Geometry: see drawing. Coordinates: mm, zero at the bounding-box minimum. Round coordinates to 2 decimals unless told otherwise and drop trailing zeros. Loops run counter-clockwise (first coordinate to the right, second up) from the corner with the lowest first, then second, coordinate; pieces in that order, holes last. Notation, with made-up numbers: (41, 39) - (86, 39) arc R25 ccw to (86, 58) - close; hole circle Ø4 at (24.5, -35). An arc over 180 degrees is marked (long way). Use CSV: the item, a comma, the result in double quotes.
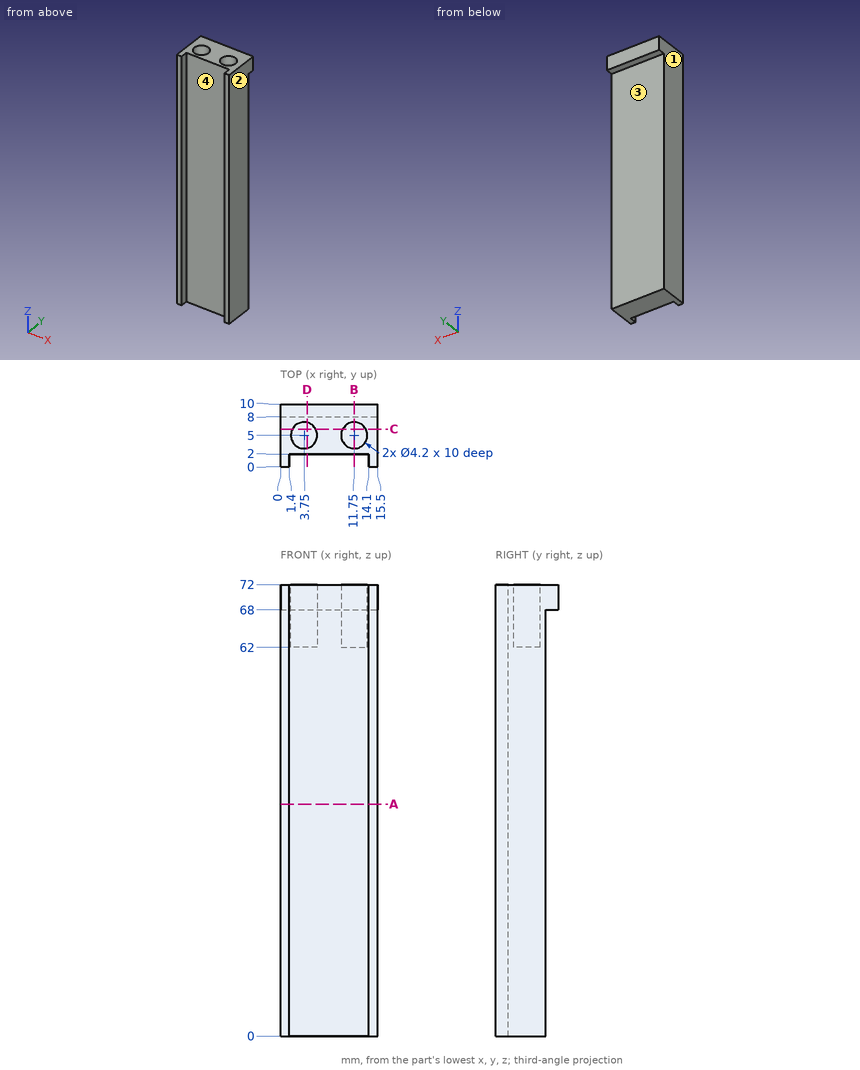
Item 1: Material intervals for line 1 (X direction, y = 0.75, z = 7); line 2 (Z direction, x = 13.25, y = 8.75); line 3 (X direction, y = 4.5, z = 65), sorted ascending.
Final values:
line 1,"x = 0 to 1.4, 14.1 to 15.5"
line 2,"z = 68 to 72"
line 3,"x = 0 to 1.71, 5.79 to 9.71, 13.79 to 15.5"
Item 2: Pin query (flat end, axial travel): P1, Ø1, axis at x = 5, y = 4.5, coming from the +Z side; P2, Ø2, axis at x = 5, z = 29, coming from the -Y side; P3, Ø0.6, axis at x = 10, y = 8.5, coming from the -Z side. Return the tip coordinate at first contact, or that it passes through.
Final values:
P1,"stops at z = 62"
P2,"stops at y = 2"
P3,"stops at z = 68"
Item 3: Section B-B on x = 11.75. Return the cut outline in (y, z).
Final values:
outline,"(2, 0) - (8, 0) - (8, 68) - (10, 68) - (10, 72) - (7.1, 72) - (7.1, 62) - (2.9, 62) - (2.9, 72) - (2, 72) - close"
Item 4: Section C-C on y = 6. Return the cut outline in (x, z), plus the area to 3 significant figures.
Final values:
outline,"(0, 0) - (15.5, 0) - (15.5, 72) - (13.6, 72) - (13.6, 62) - (9.9, 62) - (9.9, 72) - (5.6, 72) - (5.6, 62) - (1.9, 62) - (1.9, 72) - (0, 72) - close"
area,"1,040 mm²"
Item 5: Section D-D on x = 4.25. Return the cut outline in (y, z), plus the area to 3 significant figures.
Final values:
outline,"(2, 0) - (8, 0) - (8, 68) - (10, 68) - (10, 72) - (7.04, 72) - (7.04, 62) - (2.96, 62) - (2.96, 72) - (2, 72) - close"
area,"399 mm²"
Item 6: Section A-A on z = 37. Return the cut outline in (x, y), plus the area to 3 significant figures.
Final values:
outline,"(0, 0) - (1.4, 0) - (1.4, 2) - (14.1, 2) - (14.1, 0) - (15.5, 0) - (15.5, 8) - (0, 8) - close"
area,"98.6 mm²"
Item 7: Mould query, pull axis X, two halves, no side actions, for the marked faces 1, 2, 3 and 4. Classes: released by +X, released by -X, zero draft, split by the parting line, or undercut.
Final values:
face 1,"released by -X"
face 2,"released by +X"
face 3,"zero draft"
face 4,"undercut"
